from build123d import *

# Parameters (mm, degrees)
BOSS_EXTRUDE1_DEPTH       = 6.35
M3X0_5_TAPPED_HOLE1_D     = 2.5
M3X0_5_TAPPED_HOLE1_DEPTH = 6.35
F_10_CLEARANCE_HOLE1_D    = 5.1054


with BuildPart() as part:
    # Sketch1 → Boss-Extrude1 (new body)
    with BuildSketch(Plane.XY):
        with BuildLine():
            Line((1.600151217, 9.423790263), (26.200075609, 6.299395131))
            ThreePointArc((26.200075609, 6.299395131), (31.75, 0), (26.200075609, -6.299395131))
            Line((26.200075609, -6.299395131), (1.600151217, -9.423790263))
            ThreePointArc((1.600151217, -9.423790263), (0, -9.525), (-1.600151217, -9.423790263))
            Line((-1.600151217, -9.423790263), (-26.200075609, -6.299395131))
            ThreePointArc((-26.200075609, -6.299395131), (-31.75, 0), (-26.200075609, 6.299395131))
            Line((-26.200075609, 6.299395131), (-1.600151217, 9.423790263))
            ThreePointArc((-1.600151217, 9.423790263), (0, 9.525), (1.600151217, 9.423790263))
        make_face()
    extrude(amount=BOSS_EXTRUDE1_DEPTH)

    # M3x0.5 Tapped Hole1
    with Locations(Plane(origin=(0, 0, 0), x_dir=(-1, 0, 0), z_dir=(0, 0, -1))):
        with Locations((-11, 0), (11, 0)):
            Hole(M3X0_5_TAPPED_HOLE1_D / 2, depth=M3X0_5_TAPPED_HOLE1_DEPTH)

    # #10 Clearance Hole1 (through all)
    with Locations(Plane(origin=(0, 0, 0), x_dir=(-1, 0, 0), z_dir=(0, 0, -1))):
        with Locations((25.4, 0), (-25.4, 0)):
            Hole(F_10_CLEARANCE_HOLE1_D / 2)


solid = part.part
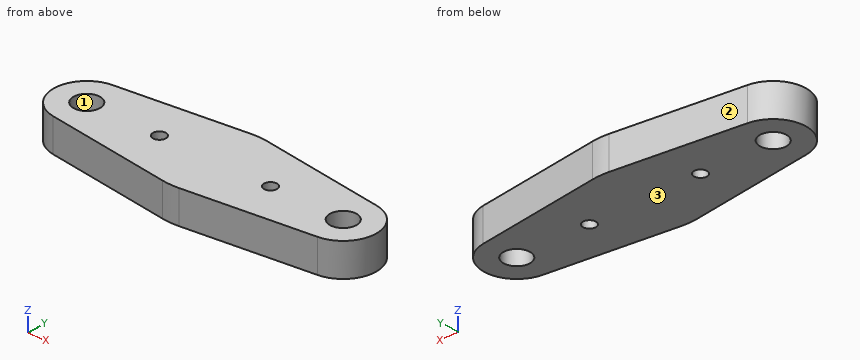
Read the model definition and answer for the solid it produces. Units are mm, in the model's axes. Face numbers are marked on the shaded views. Give positions to 0.01 mm unless a question says otherwise; leave off trailing zeros. Write each loop counter-clockwise with the first axis right and the second up, starting at its lowest first coordinate (ties: lowest second). Pieces come first, ordered by that corner, then holes. Notation, with made-up numbers: (14.25, -1) -> (65.25, -1) arc R23 cw to (65.25, 16) -> close; hole circle Ø7 at (20.25, 9.25). An arc over 180 degrees is marked (long way). Answer as a JSON object with one key per item and string values. Group by question number.
1) Find section C-C (x = 25.4). Write down the section's boundary in (y, z).
2) Each of these flat-tipped pins is pushed along its axis until it touches: P1, Ø3, axis at x = -11, y = 0, coming from the -Z side; P2, Ø2, axis at y = 4, z = 2.5, coming from the -X side; P3, Ø2, axis at y = -3.5, z = 3.5, coming from the -X side; P4, Ø3, axis at y = 4.5, z = 3.5, coming from the +X side. Where does it stop, or does it pass through?
3) Consider L1, parallel to X at y = 2, z = 3.25; L2, parallel to X at y = 0.25, z = 3.25; L3, parallel to Y at x = 26, z = 5. Determine where each line is inside the solid, lowest interval first. Write a range as from..to.
4) The mould has two halves that part along X. Classify the marked faces 1, 2 and 3: +X half, -X half, draft (parallel to the pull), parting line (faces both ways), or undercut.
5) Find section A-A (y = 0). Write down the section's boundary in (x, z).
6) Find section B-B (z = 3.75). Write down the section's boundary in (x, y) (3 decimals), and give its area (3 significant figures).
7) Find section D-D (x = 11). Write down the section's boundary in (y, z), and give its area (3 significant figures).
Values follow:
{
 "1": {"outline": "(-6.4, 0) -> (-2.55, 0) -> (-2.55, 6.35) -> (-6.4, 6.35) -> close; (2.55, 0) -> (6.4, 0) -> (6.4, 6.35) -> (2.55, 6.35) -> close"},
 "2": {"P1": "stops at z = 0", "P2": "stops at x = -31", "P3": "stops at x = -31.24", "P4": "stops at x = 31"},
 "3": {"L1": "x = -31.43..-26.99, -23.81..23.81, 26.99..31.43", "L2": "x = -31.75..-27.94, -22.86..-12.22, -9.78..9.78, 12.22..22.86, 27.94..31.75", "L3": "y = -6.32..-2.48, 2.48..6.32"},
 "4": {"face 1": "undercut", "face 2": "-X half", "face 3": "draft"},
 "5": {"outline": "(-31.75, 0) -> (-27.95, 0) -> (-27.95, 6.35) -> (-31.75, 6.35) -> close; (-22.85, 0) -> (-12.25, 0) -> (-12.25, 6.35) -> (-22.85, 6.35) -> close; (-9.75, 0) -> (9.75, 0) -> (9.75, 6.35) -> (-9.75, 6.35) -> close; (12.25, 0) -> (22.85, 0) -> (22.85, 6.35) -> (12.25, 6.35) -> close; (27.95, 0) -> (31.75, 0) -> (31.75, 6.35) -> (27.95, 6.35) -> close"},
 "6": {"outline": "(-26.2, -6.299) -> (-1.6, -9.424) arc R12.7 ccw to (1.6, -9.424) -> (26.2, -6.299) arc R6.35 ccw to (26.2, 6.299) -> (1.6, 9.424) arc R12.7 ccw to (-1.6, 9.424) -> (-26.2, 6.299) arc R6.35 ccw to start; hole circle Ø5.105 at (-25.4, 0); hole circle Ø2.5 at (-11, 0); hole circle Ø2.5 at (11, 0); hole circle Ø5.105 at (25.4, 0)", "area": "890 mm2"},
 "7": {"outline": "(-8.23, 0) -> (-1.25, 0) -> (-1.25, 6.35) -> (-8.23, 6.35) -> close; (1.25, 0) -> (8.23, 0) -> (8.23, 6.35) -> (1.25, 6.35) -> close", "area": "88.6 mm2"}
}
